```python
from build123d import *

# Parameters (mm, degrees)
FILLET_R = 1


with BuildPart() as obj1_interior:
    # Cone001 → Cone001 (revolve)
    with BuildSketch(Plane(origin=(0, 0, 2), x_dir=(1, 0, 0), z_dir=(0, -1, 0))):
        Polygon((0, 0), (13, 0), (23, 70), (0, 70), align=None)
    revolve(axis=Axis((0, 0, 2), (0, 0, 1)))


with BuildPart() as obj1:
    # Cone → Cone (revolve)
    with BuildSketch(Plane.XZ):
        Polygon((0, 0), (15, 0), (25, 70), (0, 70), align=None)
    revolve(axis=Axis((0, 0, 0), (0, 0, 1)))

    # Cut: cut obj1_interior
    add(obj1_interior.part, mode=Mode.SUBTRACT)

    # Fillet
    fillet_edges = [obj1.edges().sort_by_distance(p)[0] for p in [
        (-25, 0, 70),
        (-22.714286, 0, 70),
    ]]
    fillet(fillet_edges, radius=FILLET_R)


solid = obj1.part
```
Could you check a few things on this model? Use its own coordinates, in mm. Round coordinates to 2 decimals unless told otherwise and drop trailing zeros. Write each loop counter-clockwise with the first axis right and the second up, starting at its lowest first coordinate (ties: lowest second). Pieces come first, ordered by that corner, then holes. Notation, with made-up numbers: M 71.5,80.25 L 129.5,80.25 A24 ccw 129.5,96.25 Z; hole C -39,47.5 d7. An arc over 180 degrees is marked long. Write each question's results on one line, items separated by ' | '. Start each with the question number.
1. Imagine slicing it at A-A on x = 0. List the corners of the cut face in (y, z) for me.
2. Thinking about a two-plate mould opening in Y: for faces 1 (the face through (-4.333, -19.512, 34.911)), 2 (the face through (0, 0, 2)), 3 (the face through (0, 0, 0)), which applies, +Y half, -Y half, draft (parallel to the pull), parting line (faces both ways), or undercut?
3. I need wall thicknesses on L1, parallel to Y at x = -9.5, z = 22; L2, parallel to X at y = -6, z = 13.5; L3, parallel to X at y = 4.5, z = 18. Which ranges of each line are inside material? Lowest first, please. Write a range as from..to.
4. Imagine slicing it at C-C on z = 29. List the corners of the cut face in (x, y) for me.
5. I'm going to push flat-ended pins straight in: pin 1 Ø1 at (x, z) = (-8, 18.5) entering from -Y; pin 2 Ø10 at (y, z) = (17, 29.5) entering from -X; pin 3 Ø3 at (y, z) = (8.5, 12) entering from +X. Where does each tip first touch, or does it pass through?
6. Imagine slicing it at D-D on z = 41.5. List the corners of the cut face in (x, y) for me, and give its area (3 significant figures).
Result sheet:
1) outline: M -24.84,68.86 L -15,0 L 15,0 L 24.84,68.86 A1 ccw 23.85,70 L 23.58,70 A1 ccw 22.59,69.14 L 13,2 L -13,2 L -22.59,69.14 A1 ccw -23.58,70 L -23.85,70 A1 ccw Z
2) face 1: parting line | face 2: undercut | face 3: draft
3) L1: y = -15.46..-12.7, 12.7..15.46 | L2: x = -15.83..-13.36, 13.36..15.83 | L3: x = -16.99..-14.61, 14.61..16.99
4) outline: C 0,0 d38.29; hole C 0,0 d33.71
5) pin 1: stops at y = -15.98 | pin 2: stops at x = -15.11 | pin 3: stops at x = 15.22
6) outline: C 0,0 d41.86; hole C 0,0 d37.29 | area: 284 mm^2
